Check sheet for the modelled part. Datum: model origin and axes. Units: mm. Face numbers are marked on the shaded views. A direction names the side the tool comes from. Coordinates: 2 decimals unless noted, no trailing zeros. Write each loop counter-clockwise with the first axis right and the second up, starting at its lowest first coordinate (ties: lowest second). Pieces come first, ordered by that corner, then holes. Notation, with made-up numbers: M 20.25,11 L 42.25,11 A23 cw 42.25,34 Z; hole C -11,67.5 d7. An arc over 180 degrees is marked long. Answer as CSV lines item,"result". Start each with the question number.
Q1. Sectioned sample at B-B, the plane y = -2.5. Record the cut outline in (x, z), then the cut area to 3 significant figures.
Q2. Sectioned sample at A-A, the plane z = 11. Record the cut outline in (x, y), then the cut area to 3 significant figures.
Q3. Access from +Z, -Z, +X, -X, +Y, -Y to the whole of each face (thin tool, end or side, straight path). Record for the marked faces 1 and 2.
Q4. Sectioned sample at C-C, the plane x = 5. Record the cut outline in (y, z).
Q5. Depth check by flat-ended pin: pin 1 Ø1.6 at (y, z) = (-2.5, 11) entering from +X; pin 2 Ø8 at (x, z) = (6, -19.5) entering from -Y. Enter the tip coordinate at first touch or a pass-through.
Q6. Thickness scan on line 1 along Y through (x, z) = (0, -39); line 2 along Y through (x, z) = (16, 24); line 3 along X through (y, z) = (-1.05, -10). Record the ranges inside material, lowest first. Write a range as from..to.
from build123d import *

# Parameters (mm, degrees)
F0_W     = 3.04038
F0_H     = 103.9368
F1_DEPTH = 3.81
F2_W     = 3.175
F2_H     = 103.9368
F3_DEPTH = 2.72288
F4_W     = 0.3175
F4_H     = 51.9684
F5_DEPTH = 29.21762


with BuildPart() as f1:
    # F0 (on Front) → F1 (new body)
    with BuildSketch(Plane.XZ):
        Rectangle(F0_W, F0_H)
    extrude(amount=F1_DEPTH)

    # F2 (on face) → F3 (cut)
    with BuildSketch(Plane.YZ.offset(1.52019)):
        with Locations((-1.905, 0)):
            Rectangle(F2_W, F2_H)
    extrude(amount=-F3_DEPTH, mode=Mode.SUBTRACT)

    # F4 (on face) → F5 (join)
    with BuildSketch(Plane.YZ.offset(1.52019)):
        with Locations((-0.15875, 0)):
            Rectangle(F4_W, F4_H)
    extrude(amount=F5_DEPTH)


solid = f1.part
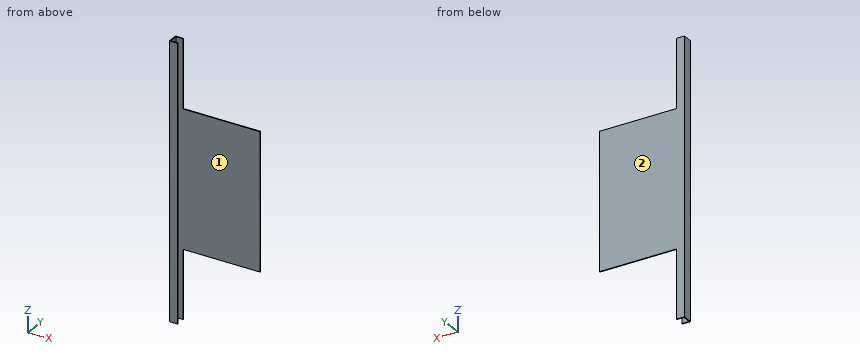
Output:
1,outline,"M -1.52,-51.97 L -1.2,-51.97 L -1.2,51.97 L -1.52,51.97 Z"
1,area,"33.0 mm^2"
2,outline,"M -1.52,-3.81 L 1.52,-3.81 L 1.52,-3.49 L -1.2,-3.49 L -1.2,-0.32 L 30.74,-0.32 L 30.74,0 L -1.52,0 Z"
2,area,"12.2 mm^2"
3,face 1,"+Z, -Z, +X"
3,face 2,"+Z, -Z, +X, -X, +Y"
4,outline,"M -0.32,-25.98 L 0,-25.98 L 0,25.98 L -0.32,25.98 Z"
5,pin 1,"stops at x = -1.2"
5,pin 2,"stops at y = -0.32"
6,line 1,"y = -3.81..-3.49, -0.32..0"
6,line 2,"y = -0.32..0"
6,line 3,"x = -1.52..-1.2"
